from build123d import *

# Parameters (mm, degrees)
SKETCH_1_W           = 30
SKETCH_1_H           = 15
EXTRUDE_1_DEPTH      = 1
EXTRUDE_2_DEPTH      = 3
EXTRUDE_2_DEPTH_BACK = 2
SKETCH_2_W           = 30
SKETCH_2_H           = 11.139726918
SKETCH_2_R           = 2
SKETCH_3_W           = 6.3
SKETCH_3_H           = 1
CUT_EXTRUDE_1_DEPTH  = 3
EXTRUDE_3_DEPTH      = 1
EXTRUDE_4_DEPTH      = 5
CUT_EXTRUDE_2_REACH  = 31.173
SKETCH_8_W           = 2.28807502
SKETCH_8_H           = 1
EXTRUDE_6_DEPTH      = 5
SKETCH_10_W          = 16.28
SKETCH_10_H          = 1.956604577
SKETCH_10_H_2        = 1.932582498
EXTRUDE_7_DEPTH      = 3
CUT_EXTRUDE_3_DEPTH  = 5


with BuildPart() as part:
    # 草图1 → 凸台-拉伸1 (new, symmetric)
    with BuildSketch(Plane.XY):
        with Locations((15, 7.5)):
            Rectangle(SKETCH_1_W, SKETCH_1_H)
    extrude(amount=EXTRUDE_1_DEPTH, both=True)

    # 草图2 → 凸台-拉伸2 (add, two sides: drawn at the far end of the back side and taken through both)
    with BuildSketch(Plane.XY.offset(1).offset(-EXTRUDE_2_DEPTH_BACK)):
        with Locations((15, -5.569863459)):
            Rectangle(SKETCH_2_W, SKETCH_2_H)
        with Locations((25, -6.6)):
            Circle(SKETCH_2_R, mode=Mode.SUBTRACT)
        with Locations((5, -6.6)):
            Circle(SKETCH_2_R, mode=Mode.SUBTRACT)
    extrude(amount=EXTRUDE_2_DEPTH + EXTRUDE_2_DEPTH_BACK)

    # 草图3 → 切除-拉伸1 (cut)
    with BuildSketch(Plane.XY.offset(4)):
        with Locations((26.85, -0.5)):
            Rectangle(SKETCH_3_W, SKETCH_3_H)
        with Locations((3.15, -0.5)):
            Rectangle(SKETCH_3_W, SKETCH_3_H)
    extrude(amount=-CUT_EXTRUDE_1_DEPTH, mode=Mode.SUBTRACT)

    # 草图4 → 凸台-拉伸3 (add)
    with BuildSketch(Plane(origin=(30, 0, 0), x_dir=(0, 0, -1), z_dir=(1, 0, 0))):
        Polygon((-1.704019465, 0), (-1.704019465, 15), (-1, 15), (1, 15), (1, -3.390976711), (-4, -3.390976711), (-4, 0), align=None)
    extrude_3 = extrude(amount=EXTRUDE_3_DEPTH)

    # 草图5 → 凸台-拉伸4 (add)
    with BuildSketch(Plane.XY.offset(4)):
        Polygon((31, -3.390976711), (30, -11.139726918), (30, -3.390976711), align=None)
    extrude_4 = extrude(amount=-EXTRUDE_4_DEPTH)

    # 镜向1: 凸台-拉伸3, 凸台-拉伸4 across plane
    add(extrude_3.mirror(Plane(origin=(15, 0, 0), x_dir=(0, 0, 1), z_dir=(1, 0, 0))))
    add(extrude_4.mirror(Plane(origin=(15, 0, 0), x_dir=(0, 0, 1), z_dir=(1, 0, 0))))

    # 草图8 → 切除-拉伸2 (cut, up to next)
    with BuildSketch(Plane.ZY.offset(-6.3), mode=Mode.PRIVATE) as cut_extrude_2_sk1:
        with Locations((2.85596249, -0.5)):
            Rectangle(SKETCH_8_W, SKETCH_8_H)
    cut_extrude_2_tool1 = extrude(cut_extrude_2_sk1.sketch, amount=-CUT_EXTRUDE_2_REACH, mode=Mode.PRIVATE) & part.part
    add(cut_extrude_2_tool1.solids().sort_by_distance((6.3, -0.5, 2.855962))[0], mode=Mode.SUBTRACT)

    # 草图9 → 凸台-拉伸6 (add)
    with BuildSketch(Plane.XY.offset(1)):
        Polygon((6.147776054, 15), (3.073888027, 15), (3.073888027, 11.936980184), (6.147776054, 11.936980184), (6.246340003, 11.936980184), (6.246340003, 11.013255946), (7.737344454, 11.013255946), (7.737344454, 15), align=None)
        Polygon((23.852223946, 15), (22.262655546, 15), (22.262655546, 11.013255946), (23.753659997, 11.013255946), (23.753659997, 11.936980184), (23.852223946, 11.936980184), (26.926111973, 11.936980184), (26.926111973, 15), align=None)
    extrude(amount=EXTRUDE_6_DEPTH)

    # 草图10 → 凸台-拉伸7 (add)
    with BuildSketch(Plane.XY.offset(1)):
        with Locations((15, 2.926222334)):
            Rectangle(SKETCH_10_W, SKETCH_10_H)
        with Locations((15, 8.136975565)):
            Rectangle(SKETCH_10_W, SKETCH_10_H_2)
    extrude(amount=EXTRUDE_7_DEPTH)

    # 草图11 → 切除-拉伸3 (cut)
    with BuildSketch(Plane.XY.offset(6)):
        Polygon((3.073888027, 11.936980184), (6.246340003, 11.936980184), (6.246340003, 11.013255946), (6.465703182, 11.013255946), (6.465703182, 12.1), (3.073888027, 12.1), align=None)
        Polygon((26.926111973, 11.936980184), (26.926111973, 12.1), (23.534296818, 12.1), (23.534296818, 11.013255946), (23.753659997, 11.013255946), (23.753659997, 11.936980184), align=None)
    extrude(amount=-CUT_EXTRUDE_3_DEPTH, mode=Mode.SUBTRACT)


solid = part.part
Part model, mm, in its own coordinate system. A direction names the side the tool comes from. Give positions to 0.01 mm unless a question says otherwise; leave off trailing zeros. Write each loop counter-clockwise with the first axis right and the second up, starting at its lowest first coordinate (ties: lowest second). Pieces come first, ordered by that corner, then holes.
1) Cut at B-B on x = 5. Write the cut outline in (y, z), then the cut area to 3 significant figures.
Resolved:
outline: (-11.14, -1) - (-8.6, -1) - (-8.6, 4) - (-11.14, 4) - close; (-4.6, -1) - (15, -1) - (15, 6) - (12.1, 6) - (12.1, 1) - (-1, 1) - (-1, 4) - (-4.6, 4) - close
area: 77.2 mm2
2) Pin check, flat tips, straight feed: pin 1 (1.1 mm diameter, centred on x = -0.5, y = 9.5, fed in from +Z); pin 2 (0.6 mm diameter, centred on x = 23, z = 4.5, fed in from -Y); pin 3 (2 mm diameter, centred on y = 8.5, z = 3, fed in from -X); pin 4 (3.5 mm diameter, centred on x = 16.5, z = 2.5, fed in from +Y). Stop position of each tip, or through.
Resolved:
pin 1: stops at z = 1.7
pin 2: stops at y = 11.01
pin 3: stops at x = 6.86
pin 4: stops at y = 15
3) Two-plate mould, pull along Y, no slides. Class faces 1 (the face through (7, 11.013, 3)), 2 (the face through (30.507, -7.211, 1.535)), 3 (the face through (-0.5, 7.4, 1.704)): released by +Y, released by -Y, zero draft, split by the parting line, or undercut.
Resolved:
face 1: undercut
face 2: released by -Y
face 3: zero draft
4) Cut at C-C on x = 17. Write the cut outline in (y, z), then the cut area to 3 significant figures.
Resolved:
outline: (-11.14, -1) - (15, -1) - (15, 1) - (9.1, 1) - (9.1, 4) - (7.17, 4) - (7.17, 1) - (3.9, 1) - (3.9, 4) - (1.95, 4) - (1.95, 1) - (0, 1) - (0, 1.71) - (-1, 1.71) - (-1, 4) - (-11.14, 4) - close
area: 95.1 mm2
5) Which spindle directions (+Z, -Z, +X, -X, +Y, -Y) get a long thin tool onto all of the face, cutting with end or side? Do faces 4 (the face through (15, 1.948, 2)), 5 (the face through (30.5, 7.4, 1.704)), 6 (the face through (15, -5, 4)). Say none if no direction does.
Resolved:
face 4: +Z
face 5: +Z, +X, +Y
face 6: +Z, +X, -X, -Y
6) Cut at D-D on z = -0.5. Write the cut outline in (x, y).
Resolved:
outline: (-1, -3.39) - (0, -11.14) - (30, -11.14) - (31, -3.39) - (31, 15) - (-1, 15) - close; hole circle Ø4 at (5, -6.6); hole circle Ø4 at (25, -6.6)
7) Probe L1, parallel to Y at x = 10, z = 2; L2, parallel to Y at x = 5, z = 1.9; L3, parallel to X at y = 12.75, z = 2.25. List the from-to ranges inside material, lowest first.
Resolved:
L1: y = -11.14 to -1, 1.95 to 3.9, 7.17 to 9.1
L2: y = -11.14 to -8.6, -4.6 to -1, 12.1 to 15
L3: x = 3.07 to 7.74, 22.26 to 26.93
8) Cut at A-A on z = 4.5. Write the cut outline in (x, y).
Resolved:
outline: (3.07, 12.1) - (6.47, 12.1) - (6.47, 11.01) - (7.74, 11.01) - (7.74, 15) - (3.07, 15) - close; (22.26, 11.01) - (23.53, 11.01) - (23.53, 12.1) - (26.93, 12.1) - (26.93, 15) - (22.26, 15) - close
